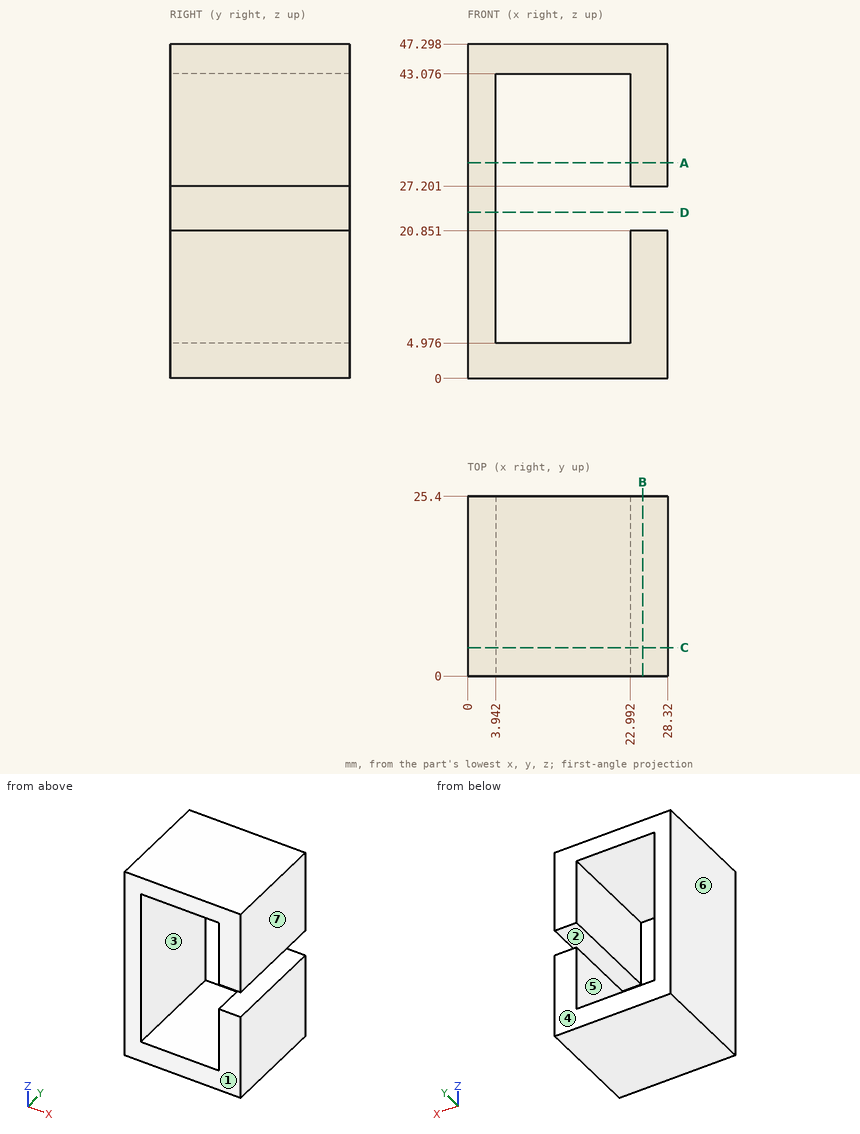
Part print with two shaded views. Sizes in mm from the minimum x, y, z corner. A direction names the side the tool comes from. Coordinates: 2 decimals unless noted, no trailing zeros. Order: outer loops, then holes, each group sorted by start corner. A loop starts at its lowest first (then second) coordinate and runs counter-clockwise, first axis right, second up. Notation, with made-up numbers: M 0,-30 L 16,-30 A15 ccw 16,-19 Z; hole C 81.5,-36.5 d9. An arc over 180 degrees is marked long. Use a Markdown table: item, result.
(1) Cut at B-B on x = 24.75. Write the cut outline in (y, z).
A:
| item | result |
|---|---|
| outline | M 0,0 L 25.4,0 L 25.4,20.85 L 0,20.85 Z; M 0,27.2 L 25.4,27.2 L 25.4,47.3 L 0,47.3 Z |
(2) Pull direction X, two halves, no side cores. Call the marked faces 4, 5, 6 and 7: released by +X, released by -X, zero draft, split by the parting line, or undercut.
A:
| item | result |
|---|---|
| face 4 | zero draft |
| face 5 | undercut |
| face 6 | released by -X |
| face 7 | released by +X |
(3) Cut at C-C on y = 4. Write the cut outline in (x, z), then the cut area to 3 significant figures.
A:
| item | result |
|---|---|
| outline | M 0,0 L 28.32,0 L 28.32,20.85 L 22.99,20.85 L 22.99,4.98 L 3.94,4.98 L 3.94,43.08 L 22.99,43.08 L 22.99,27.2 L 28.32,27.2 L 28.32,47.3 L 0,47.3 Z |
| area | 580 mm^2 |
(4) Cut at D-D on z = 23.5. Write the cut outline in (x, y), then the cut area to 3 significant figures.
A:
| item | result |
|---|---|
| outline | M 0,0 L 3.94,0 L 3.94,25.4 L 0,25.4 Z |
| area | 100 mm^2 |
(5) Tool access for the marked faces 1, 2 and 3: list every direction of +Z, -Z, +X, -X, +Y, -Y with a clear straight run to the whole face (end or side of a thin tool).
A:
| item | result |
|---|---|
| face 1 | +Z, -Z, +X, -X, -Y |
| face 2 | +X, +Y, -Y |
| face 3 | +Y, -Y |
(6) Probe L1, parallel to X at y = 21.5, z = 39; L2, parallel to Z at x = 14.25, y = 5.75; L3, parallel to X at y = 10.25, z = 27. List the from-to ranges inside material, lowest first.
A:
| item | result |
|---|---|
| L1 | x = 0 to 3.94, 22.99 to 28.32 |
| L2 | z = 0 to 4.98, 43.08 to 47.3 |
| L3 | x = 0 to 3.94 |
(7) Cut at A-A on z = 30.5. Write the cut outline in (x, y).
A:
| item | result |
|---|---|
| outline | M 0,0 L 3.94,0 L 3.94,25.4 L 0,25.4 Z; M 22.99,0 L 28.32,0 L 28.32,25.4 L 22.99,25.4 Z |
